Here's how the part is built. I have some questions about the finished solid (model axes, mm). Face numbers are marked on the shaded views. A direction names the side the tool comes from. Round coordinates to 2 decimals unless told otherwise and drop trailing zeros. Write each loop counter-clockwise with the first axis right and the second up, starting at its lowest first coordinate (ties: lowest second). Pieces come first, ordered by that corner, then holes. Notation, with made-up numbers: (-29.75, 16.5) - (10.25, 16.5) arc R22 cw to (10.25, 28.5) - close; hole circle Ø9 at (-13.5, -37). An arc over 180 degrees is marked (long way). Write item = value, one per line. Start each with the question number.
Item 1: If we section it at C-C (x = 6): Please give me the cut outline in (y, z).
Item 2: If we section it at B-B (y = 2.5): Please give me the cut outline in (x, z).
Item 3: If we section it at D-D (z = 14): Give the number of separate pieces and of enclosed holes in the cut face, and give its area (3 significant figures).
Item 4: Thinking about a two-plate mould opening in Z: for the marked faces 3, 4 and 5, which applies, pulls with the +Z half, pulls with the -Z half, needs draft (parallel to the pull), parting line crosses it, or undercut?
Item 5: For P1, Ø6, axis at x = -9.5, z = -11, coming from the +Y side; P2, Ø4, axis at x = -14, y = 2, coming from the +Z side; P3, Ø2, axis at x = -7, z = 0.5, coming from the -Y side, each with a flat end and sliding along its axis, tell me the tip position at first contact or that it passes through.
Item 6: Which directions (+Z, -Z, +X, -X, +Y, -Y) give clear straight access to the entire face, cutting with the end or side of a thin tool? Please do the marked faces 1 and 2.
Item 7: If I drill on line 1 along X through (y, z) = (-3.5, 0); line 2 along Y through (x, z) = (16.5, 6.5); line 3 along Y through (x, z) = (7.5, -0.5), over which ranges is the centre line in solid material (lowest first)? Write a range as [from, to].
Item 8: If we section it at A-A (x = 0): Please give me the cut outline in (y, z), and give its area (3 significant figures).
```python
from build123d import *

# Parameters (mm, degrees)
SKETCH1_R           = 1.55
BOSS_EXTRUDE1_DEPTH = 1.5
SKETCH2_R           = 10.5
BOSS_EXTRUDE2_DEPTH = 3
SKETCH3_R           = 5
BOSS_EXTRUDE3_DEPTH = 5
SKETCH4_R           = 2.5
CUT_EXTRUDE1_DEPTH  = 28.207535721
CHAMFER1_SIZE       = 0.5


with BuildPart() as part:
    # Sketch1 → Boss-Extrude1 (new body)
    with BuildSketch(Plane(origin=(0, 0, 0), x_dir=(1, 0, 0), z_dir=(0, 1, 0))):
        with BuildLine():
            Line((-8.485281374, 17), (8.485281374, 17))
            ThreePointArc((8.485281374, 17), (19, 0), (8.485281374, -17))
            Line((8.485281374, -17), (-8.485281374, -17))
            ThreePointArc((-8.485281374, -17), (-19, 0), (-8.485281374, 17))
        make_face()
        with Locations(Location((-16, 0, 0), (0, 0, 270))):
            Circle(SKETCH1_R, mode=Mode.SUBTRACT)
        with Locations(Location((-8, 13.856406461, 0), (0, 0, 270))):
            Circle(SKETCH1_R, mode=Mode.SUBTRACT)
        with Locations(Location((8, 13.856406461, 0), (0, 0, 270))):
            Circle(SKETCH1_R, mode=Mode.SUBTRACT)
        with Locations(Location((16, 0, 0), (0, 0, 270))):
            Circle(SKETCH1_R, mode=Mode.SUBTRACT)
        with Locations(Location((8, -13.856406461, 0), (0, 0, 270))):
            Circle(SKETCH1_R, mode=Mode.SUBTRACT)
        with Locations(Location((-8, -13.856406461, 0), (0, 0, 270))):
            Circle(SKETCH1_R, mode=Mode.SUBTRACT)
    extrude(amount=BOSS_EXTRUDE1_DEPTH)

    # Sketch2 → Boss-Extrude2 (add)
    with BuildSketch(Plane(origin=(0, 1.5, 0), x_dir=(1, 0, 0), z_dir=(0, 1, 0))):
        with Locations(Location((0, 0, 0), (0, 0, 270))):
            Circle(SKETCH2_R)
    extrude(amount=BOSS_EXTRUDE2_DEPTH)

    # Sketch3 → Boss-Extrude3 (add)
    with BuildSketch(Plane.XZ):
        with Locations(Location((0, 0, 0), (0, 0, 270))):
            Circle(SKETCH3_R)
    extrude(amount=BOSS_EXTRUDE3_DEPTH)

    # Sketch4 → Cut-Extrude1 (cut, through all)
    with BuildSketch(Plane(origin=(0, 4.5, 0), x_dir=(1, 0, 0), z_dir=(0, 1, 0))):
        with Locations(Location((0, 0, 0), (0, 0, 270))):
            Circle(SKETCH4_R)
    extrude(amount=-CUT_EXTRUDE1_DEPTH, mode=Mode.SUBTRACT)

    # Chamfer1
    chamfer1_edges = [part.edges().sort_by_distance(p)[0] for p in [
        (-19, 1.5, 0),
        (0, -5, 5),
        (19, 1.5, 0),
        (0, -5, -2.5),
        (-19, 0, 0),
        (19, 0, 0),
    ]]
    chamfer(chamfer1_edges, length=CHAMFER1_SIZE)


solid = part.part
```
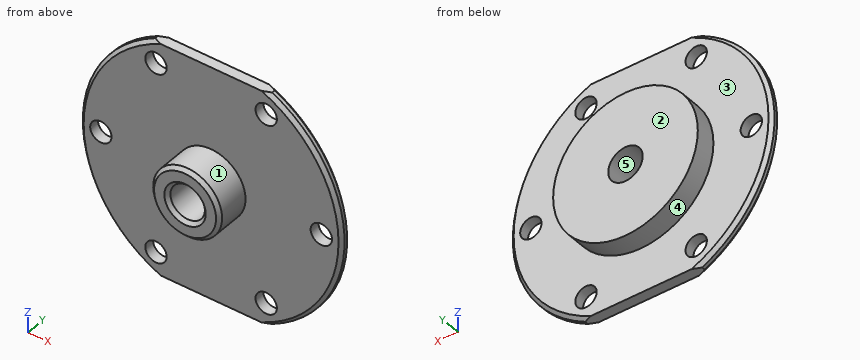
Reply:
q1.outline = (0, -17) - (1.5, -17) - (1.5, -8.62) - (4.5, -8.62) - (4.5, 8.62) - (1.5, 8.62) - (1.5, 17) - (0, 17) - close
q2.outline = circle Ø21 at (0, 0); hole circle Ø5 at (0, 0)
q3.separate_pieces = 3
q3.enclosed_holes = 0
q3.area = 28.5 mm2
q4.face_3 = needs draft
q4.face_4 = parting line crosses it
q4.face_5 = undercut
q5.P1 = 1.5
q5.P2 = 14.51
q5.P3 = 0
q6.face_1 = -Y
q6.face_2 = +Z, -Z, +X, -X, +Y
q7.line_1 = [-5, -2.5], [2.5, 5]
q7.line_2 = [0, 1.5]
q7.line_3 = [0, 4.5]
q8.outline = (-5, -4.5) - (-4.5, -5) - (0, -5) - (0, -17) - (1.5, -17) - (1.5, -10.5) - (4.5, -10.5) - (4.5, -2.5) - (-4.5, -2.5) - (-5, -3) - close; (-5, 3) - (-4.5, 2.5) - (4.5, 2.5) - (4.5, 10.5) - (1.5, 10.5) - (1.5, 17) - (0, 17) - (0, 5) - (-4.5, 5) - (-5, 4.5) - close
q8.area = 116 mm2
